```python
from build123d import *

# Parameters (mm, degrees)
F0_W     = 182.7391684055
F0_H     = 124.0453347564
F0_W_2   = 159.4799607992
F0_H_2   = 92.0757874846
F1_DEPTH = 101.6
F2_W     = 103.849850595
F2_H     = 51.4723447323
F3_DEPTH = 1270
F4_R     = 15.0246313373
F5_DEPTH = 1270


with BuildPart() as f1:
    # F0 (on Top) → F1 (new body)
    with BuildSketch(Plane.XY):
        Rectangle(F0_W, F0_H)
        Rectangle(F0_W_2, F0_H_2, mode=Mode.SUBTRACT)
    extrude(amount=F1_DEPTH)

    # F2 (on face) → F3 (cut)
    with BuildSketch(Plane.XZ.offset(62.0226673782)):
        with Locations((0, 75.8638276339)):
            Rectangle(F2_W, F2_H)
    extrude(amount=-F3_DEPTH, mode=Mode.SUBTRACT)

    # F4 (on face) → F5 (cut)
    with BuildSketch(Plane.YZ.offset(91.3695842028)):
        with Locations((0, 50.8573576808)):
            Circle(F4_R)
    extrude(amount=-F5_DEPTH, mode=Mode.SUBTRACT)


solid = f1.part
```
For this review, take the finished solid that the model builds, in its own axes (mm). A direction names the side the tool comes from. Coordinates: 2 decimals unless noted, no trailing zeros. Order: outer loops, then holes, each group sorted by start corner. A loop starts at its lowest first (then second) coordinate and runs counter-clockwise, first axis right, second up. Notation, with made-up numbers: (-3.75, -2.75) - (44.25, -2.75) arc R13 ccw to (44.25, 15.25) - close; hole circle Ø1 at (0, -37.75). An arc over 180 degrees is marked (long way). Answer as a JSON object with one key per item and string values. Group by question number.
1. Clearance check with flat-ended pins moving along their axes: P1, Ø18, axis at y = 0, z = 50.86, coming from the +X side; P2, Ø5, axis at x = 5.5, y = -57.5, coming from the +Z side. State where each tip first meets the part, or that it passes through.
2. For probe 1 along X at (y, z) = (-19, 37.5); probe 2 along Z at (x, y) = (84, 0); probe 3 along X at (y, z) = (-50.5, 84), list the stretches that pass through material, from the lowest coordinate up.
3. We need section C-C on y = 27. State the section outline as (x, z) points, then the cut area to 3 significant figures.
4. For faces 4 (the flat face through (51.925, 54, 76)), 5 (the flat face through (-1, -62.023, 39)), 6 (the flat face through (-1, -46.038, 39)), list the 3-axis set-ups (+Z, -Z, +X, -X, +Y, -Y) from which the entire face can be reached by the end or side of a thin tool; tool diameter is ignored.
5. We need section D-D on z = 18. State the section outline as (x, y) points, then the cut area to 3 significant figures.
6. The part is to be moulded in two halves that separate along X. For faces 1 (the flat face through (-79.74, -11, 39)), 2 (the flat face through (-91.37, 13, 61)), 3 (the cylindrical face through (-85.5, -3.3, 36.2)), say which applies: pulls with the +X half, pulls with the -X half, needs draft (parallel to the pull), parting line crosses it, or undercut.
7. We need section A-A on x = 0.5. State the section outline as (y, z) points.
8. We need section B-B on z = 71. State the section outline as (x, y) points.
Final values:
{
 "1": {"P1": "through", "P2": "z = 50.13"},
 "2": {"probe 1": "-91.37 to -79.74, 79.74 to 91.37", "probe 2": "0 to 35.83, 65.88 to 101.6", "probe 3": "-91.37 to -51.92, 51.92 to 91.37"},
 "3": {"outline": "(-91.37, 0) - (-79.74, 0) - (-79.74, 101.6) - (-91.37, 101.6) - close; (79.74, 0) - (91.37, 0) - (91.37, 101.6) - (79.74, 101.6) - close", "area": "2,360 mm²"},
 "4": {"face 4": "+Z, +Y, -Y", "face 5": "+Z, -Z, +X, -X, -Y", "face 6": "+Z, -Z"},
 "5": {"outline": "(-91.37, -62.02) - (91.37, -62.02) - (91.37, 62.02) - (-91.37, 62.02) - close; hole (-79.74, -46.04) - (79.74, -46.04) - (79.74, 46.04) - (-79.74, 46.04) - close", "area": "7,980 mm²"},
 "6": {"face 1": "undercut", "face 2": "pulls with the -X half", "face 3": "needs draft"},
 "7": {"outline": "(-62.02, 0) - (-46.04, 0) - (-46.04, 50.13) - (-62.02, 50.13) - close; (46.04, 0) - (62.02, 0) - (62.02, 50.13) - (46.04, 50.13) - close"},
 "8": {"outline": "(-91.37, -62.02) - (-51.92, -62.02) - (-51.92, -46.04) - (-79.74, -46.04) - (-79.74, 46.04) - (-51.92, 46.04) - (-51.92, 62.02) - (-91.37, 62.02) - close; (51.92, -62.02) - (91.37, -62.02) - (91.37, 62.02) - (51.92, 62.02) - (51.92, 46.04) - (79.74, 46.04) - (79.74, -46.04) - (51.92, -46.04) - close"}
}
